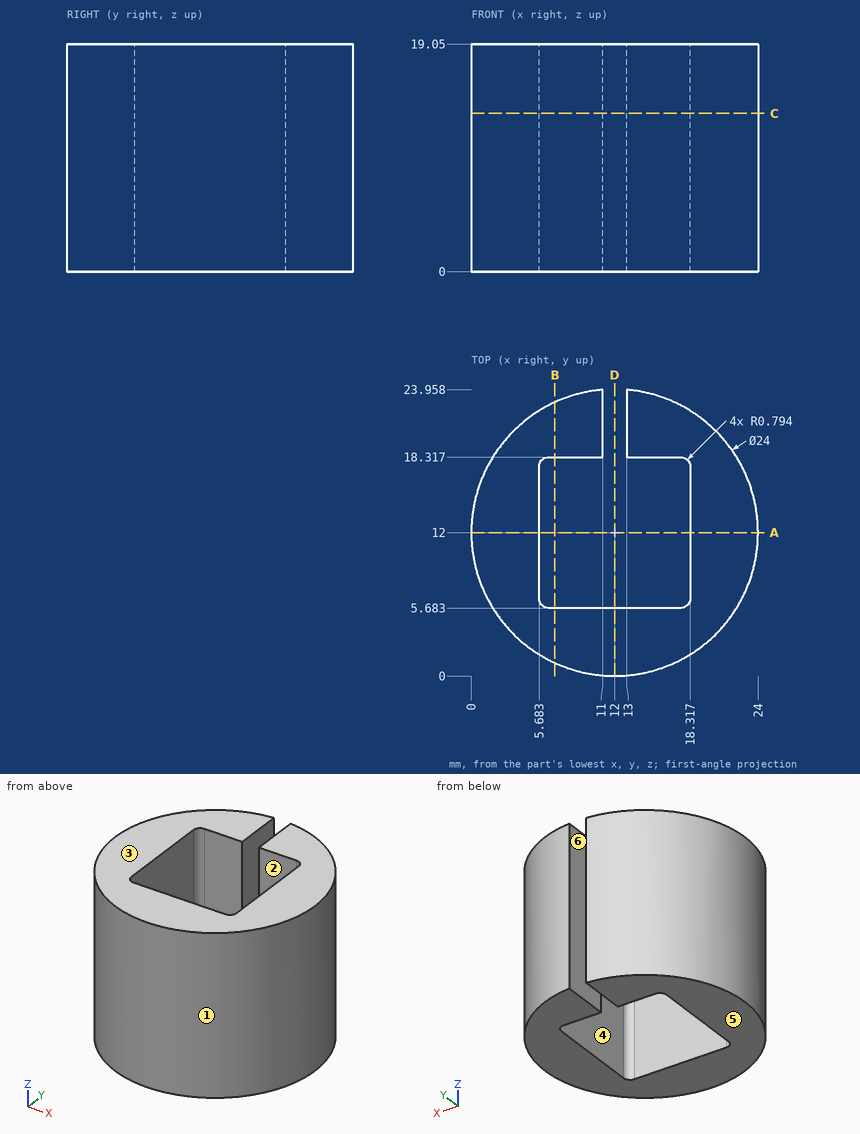
Here's the drawing with two shaded views (mm, measured from the low corner). I have some questions. A direction names the side the tool comes from. Coordinates: 2 decimals unless noted, no trailing zeros. Order: outer loops, then holes, each group sorted by start corner. A loop starts at its lowest first (then second) coordinate and runs counter-clockwise, first axis right, second up.
Q1. Will these pins go through, and if not, where does the flat tip stop? pin 1 (1.5 mm diameter, centred on y = 13.5, z = 15, fed in from +X); pin 2 (2.5 mm diameter, centred on x = 15, z = 9, fed in from -Y); pin 3 (8 mm diameter, centred on x = 19, z = 5, fed in from +Y); pin 4 (6 mm diameter, centred on x = 12, y = 16.5, fed in from +Z).
Q2. Which directions (+Z, -Z, +X, -X, +Y, -Y) give clear straight access to the entire face, cutting with the end or side of a thin tool? Please do the marked faces 4, 5 and 6.
Q3. Suppose I cut it at D-D on x = 12. Please give me the cut outline in (y, z), and give its area (3 significant figures).
Q4. Suppose I cut it at C-C on z = 13.25. Please give me the cut outline in (x, y), and give its area (3 significant figures).
Q5. Thinking about a two-plate mould opening in X: for the marked faces 1, 2 and 3, which applies, released by +X, released by -X, zero draft, split by the parting line, or undercut?
Q6. Suppose I cut it at A-A on y = 12. Please give me the cut outline in (x, z).
Q7. Suppose I cut it at B-B on x = 7. Please give me the cut outline in (y, z), and give its area (3 significant figures).
Q8. Please list where these lines run through material, in increasing order: L1, parallel to X at y = 15.5, z = 8.75; L2, parallel to Y at x = 7.25, z = 5.5; L3, parallel to X at y = 19, z = 1.5.
Answer:
1. pin 1: stops at x = 23.98
1. pin 2: stops at y = 0.13
1. pin 3: stops at y = 23.62
1. pin 4: stops at z = 19.05
2. face 4: +Z, -Z
2. face 5: -Z, +X, -X, +Y, -Y
2. face 6: +Z, -Z, +Y
3. outline: (0, 0) - (5.68, 0) - (5.68, 19.05) - (0, 19.05) - close
3. area: 108 mm2
4. outline: (5.68, 6.48) - (5.68, 17.52) arc R0.79 cw to (6.48, 18.32) - (11, 18.32) - (11, 23.96) arc R12 ccw (long way) to (13, 23.96) - (13, 18.32) - (17.52, 18.32) arc R0.79 cw to (18.32, 17.52) - (18.32, 6.48) arc R0.79 cw to (17.52, 5.68) - (6.48, 5.68) arc R0.79 cw to start
4. area: 282 mm2
5. face 1: split by the parting line
5. face 2: undercut
5. face 3: zero draft
6. outline: (0, 0) - (5.68, 0) - (5.68, 19.05) - (0, 19.05) - close; (18.32, 0) - (24, 0) - (24, 19.05) - (18.32, 19.05) - close
7. outline: (1.09, 0) - (5.68, 0) - (5.68, 19.05) - (1.09, 19.05) - close; (18.32, 0) - (22.91, 0) - (22.91, 19.05) - (18.32, 19.05) - close
7. area: 175 mm2
8. L1: x = 0.52 to 5.68, 18.32 to 23.48
8. L2: y = 0.98 to 5.68, 18.32 to 23.02
8. L3: x = 2.25 to 11, 13 to 21.75
